Source: CAD feature listing. Evaluate the final solid. Frame: model axes, mm. Face numbers are marked on the shaded views. Coordinates: 2 decimals unless noted, no trailing zeros. Order: outer loops, then holes, each group sorted by start corner. A loop starts at its lowest first (then second) coordinate and runs counter-clockwise, first axis right, second up. Notation, with made-up numbers: (76.25, -31) - (120.25, -31) arc R20 cw to (120.25, -15) - close; hole circle Ø7 at (27, 7). An arc over 180 degrees is marked (long way). One line per question, with ' | ' between items. Start each with the question number.
(1) Contact query for flat-ended pins moving along their axis: P1, Ø13.5, axis at x = 0, y = 30, coming from the -Z side; P2, Ø15.5, axis at x = 0, y = 30, coming from the +Z side; P3, Ø5.5, axis at x = 40.5, z = 47.5, coming from the +Y side. Output: stop coordinate, or through.
(2) Section C-C (y = 30). Return the cut outline in (x, z) (3 decimals).
(3) Line query: line 1 along Y through (x, z) = (0, 11.55) (3 decimals); line 2 along Y through (x, z) = (0, 6); line 3 along Y through (x, z) = (19, 20). Output: solid intervals per line, ascending.
(4) Section B-B (x = 0). Return the cut outline in (y, z) (3 decimals).
(5) Section A-A (z = 2). Return the cut outline in (x, y), then the cut area to 3 significant figures.
(6) Draft query along Z for the marked faces 1, 2 and 3. Return one class per face: +Z half, -Z half, draft (parallel to the pull), parting line (faces both ways), or undercut.
(7) Section D-D (x = -16.5). Return the cut outline in (y, z).
Autodesk Inventor part; units mm, degrees
ref_plane "Work Plane3" through (36.4952, -2.5, 53.75) normal (0.866, 0, 0.5) x (0, 1, 0)
ref_plane "YZ Plane" through (0, 0, 0) normal (1, 0, 0) x (0, 1, 0)
ref_plane "XZ Plane" through (0, 0, 0) normal (0, 1, 0) x (-1, 0, 0)
sketch "Sketch1" plane through (0, 0, 0) normal (0, 0, 1) x (1, 0, 0)
  circle A0 centre (0, 30) radius 8.525
  circle A1 centre (0, 30) radius 6
  arc A2 (-30, 0) -> (-15.1068, 13.2135) centre (-30, 15) ccw
  arc A3 (15.1068, 13.2135) -> (30, 0) centre (30, 15) ccw
  arc A4 (12.9075, 31.5483) -> (-12.9075, 31.5483) centre (0, 30) ccw
  line L0 (-12.9075, 31.5483) -> (-15.1068, 13.2135)
  line L1 (12.9075, 31.5483) -> (15.1068, 13.2135)
  line L2 (30, 0) -> (-30, 0)
  line L3 (-30, 0) -> (-30, -2.5)
  line L4 (-30, -2.5) -> (30, -2.5)
  line L5 (30, -2.5) -> (30, 0)
  point P0 (0, 0)
  point P1 (0, 0)
  dimension "d2" = 17.05
  dimension "d3" = 12
  dimension "d9" = 30
  dimension "d12" = 13
  dimension "d15" = 15
  dimension "d16" = 60
  dimension "d17" = 2.5
extrude "Extrusion3" add sketch "Sketch1" along normal mid plane 30 contours A2 L0 A4 L1 A3 L2
extrude "Extrusion4" add sketch "Sketch1" along normal mid plane 20 contours A0
extrude "Extrusion5" add sketch "Sketch1" against normal blind 15 contours L2 L5 L4 L3
extrude "Extrusion6" add sketch "Sketch1" along normal blind 50 contours L2 L5 L4 L3
ref_plane "Work Plane1" through (30, -2.5, 50) normal (0.866, 0, 0.5) x (0, 1, 0)
ref_plane "Work Plane3" through (36.4952, -2.5, 53.75) normal (0.866, 0, 0.5) x (0, 1, 0)
sketch "Sketch5" plane through (36.4952, -2.5, 53.75) normal (0.866, 0, 0.5) x (0, 1, 0)
  line L0 (2.5, -30.3109) -> (2.5, -18.3109) construction
  circle A0 centre (10.5, -12.1087) radius 5.35
  circle A1 centre (10.5, -12.1087) radius 7.3 construction
  line L1 (2.5, -18.3109) -> (6.65, -18.3109)
  line L2 (6.65, -18.3109) -> (6.65, -5.9065)
  line L3 (6.65, -5.9065) -> (2.5, -5.9065)
  line L4 (2.5, -5.9065) -> (2.5, -18.3109)
  point P0 (6.65, -15.8235)
  point P1 (6.65, -8.3938)
  dimension "d46" = 12
  dimension "d47" = 10.7
  dimension "d48" = 14.6
  dimension "d49" = 8
  dimension "d51" = 1.5
extrude "Extrusion9" add sketch "Sketch5" along normal mid plane 5.5 contours A0 L2 L1 L4 L3
sketch "Sketch6" plane through (30, -2.5, -15) normal (1, 0, 0) x (0, 0, -1)
  line L0 (0, 0) -> (-65, 0)
  line L1 (0, 2.5) -> (0, 0)
  line L2 (0, 2.5) -> (-30, 2.5)
  line L3 (-30, 2.5) -> (-65, 2.5)
  line L4 (-65, 0) -> (-65, 2.5)
  point P0 (-15, 2.5)
extrude "Extrusion10" add sketch "Sketch6" along normal blind 18
sketch "Sketch7" plane through (-30, 0, 15) normal (0, 1, 0) x (1, 0, 0)
  line L0 (0, 30) -> (0, -35)
  arc A0 (69.1673, -35) -> (0, 0) centre (0, -85.8445) ccw
  line L1 (0, -35) -> (78, -35)
  line L2 (0, 0) -> (60, 0)
  arc A1 (60, 30) -> (78, -24.2242) centre (150.6739, 30) ccw
  line L3 (60, 30) -> (60, 0)
  line L4 (78, 30) -> (78, -35)
  line L5 (60, 30) -> (78, 30)
  point P0 (30, 15)
  point P1 (67.0668, -32.2599)
  point P2 (78.0322, -24.2673)
extrude "Extrusion11" cut sketch "Sketch7" against normal through all contours A0 L1 L0 | L5 L4 A1
properties part number "Support"
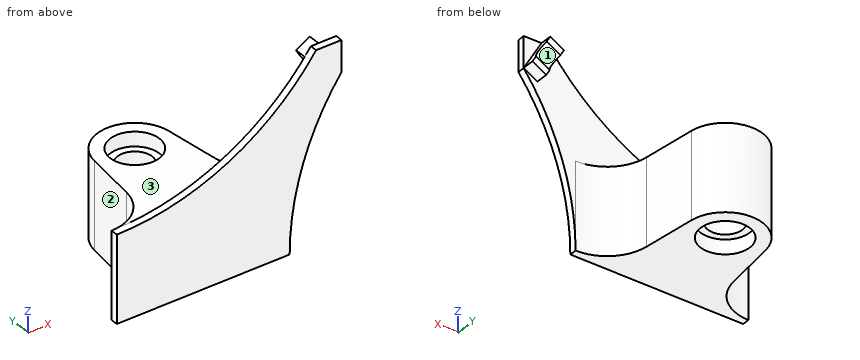
Response values:
1) P1: stops at z = -10 | P2: stops at z = 10 | P3: stops at y = 4.15
2) outline: (-13.093, -15) - (-8.525, -15) - (-8.525, -10) - (-6, -10) - (-6, 10) - (-8.525, 10) - (-8.525, 15) - (-13.093, 15) - close; (6, -10) - (8.525, -10) - (8.525, -15) - (13.093, -15) - (13.093, 15) - (8.525, 15) - (8.525, 10) - (6, 10) - close
3) line 1: y = -2.5 to 21.475, 38.525 to 43 | line 2: y = -2.5 to 24, 36 to 43 | line 3: y = -2.5 to 0
4) outline: (-2.5, -15) - (21.475, -15) - (21.475, -10) - (24, -10) - (24, 10) - (21.475, 10) - (21.475, 15) - (0, 15) - (0, 20.413) - (-2.5, 20.413) - close; (36, -10) - (38.525, -10) - (38.525, -15) - (43, -15) - (43, 15) - (38.525, 15) - (38.525, 10) - (36, 10) - close
5) outline: (-30, -2.5) - (31.61, -2.5) - (31.61, 0) - (30, 0) arc R15 cw to (15.11, 13.21) - (12.91, 31.55) arc R13 ccw to (-12.91, 31.55) - (-15.11, 13.21) arc R15 cw to (-30, 0) - close; hole circle Ø12 at (0, 30) | area: 1,270 mm²
6) face 1: undercut | face 2: draft | face 3: +Z half
7) outline: (-2.5, -15) - (8.46, -15) - (8.46, 15) - (0, 15) - (0, 16.07) - (-2.5, 16.07) - close
